Geometry: see drawing. Coordinates: mm, zero at the bounding-box minimum. A direction names the side the tool comes from. Round coordinates to 2 decimals unless told otherwise and drop trailing zeros. Order: outer loops, then holes, each group sorted by start corner. A loop starts at its lowest first (then second) coordinate and runs counter-clockwise, first axis right, second up. Notation, with made-up numbers: (31, -31.75) - (74, -31.75) arc R11 ccw to (74, -16.75) - close; hole circle Ø1 at (56.25, 22.5). An arc over 180 degrees is marked (long way). Put each result on its own line as item: value. Start each with the question number.
1) Section B-B on y = 9.25. Output: boundary loops of the cut face in (x, z) (1 decimal), then the cut area to 3 significant figures.
2) Mould query, pull axis X, two halves, no side actions, for the marked faces 6, 7 and 8. Classes: +X half, -X half, draft (parallel to the pull), parting line (faces both ways), or undercut.
3) Contact query for flat-ended pins moving along their axis: P1, Ø11, axis at x = 5.5, z = 24.5, coming from the +Y side; P2, Ø1, axis at y = 16, z = 28.5, coming from the -X side; P3, Ø7.5, axis at x = 8, y = 6.5, coming from the -Z side. Output: stop coordinate, or through.
4) Line query: probe 1 along X at (y, z) = (4.35, 25.6); probe 2 along X at (y, z) = (14, 48.5); probe 3 along Z at (x, y) = (81, 2.4). Output: solid intervals per line, ascending. Write a range as [from, to].
5) Section A-A on z = 30. Output: boundary loops of the cut face in (x, y).
6) Access query for the marked faces 1, 2, 3, 4 and 5. Directions: +Z, -Z, +X, -X, +Y, -Y. A direction counts if a zero-diameter tool reaches every point of the face in a straight line with its end or side. Return the directions, or none.
7) Section C-C on y = 21.75. Output: boundary loops of the cut face in (x, z).
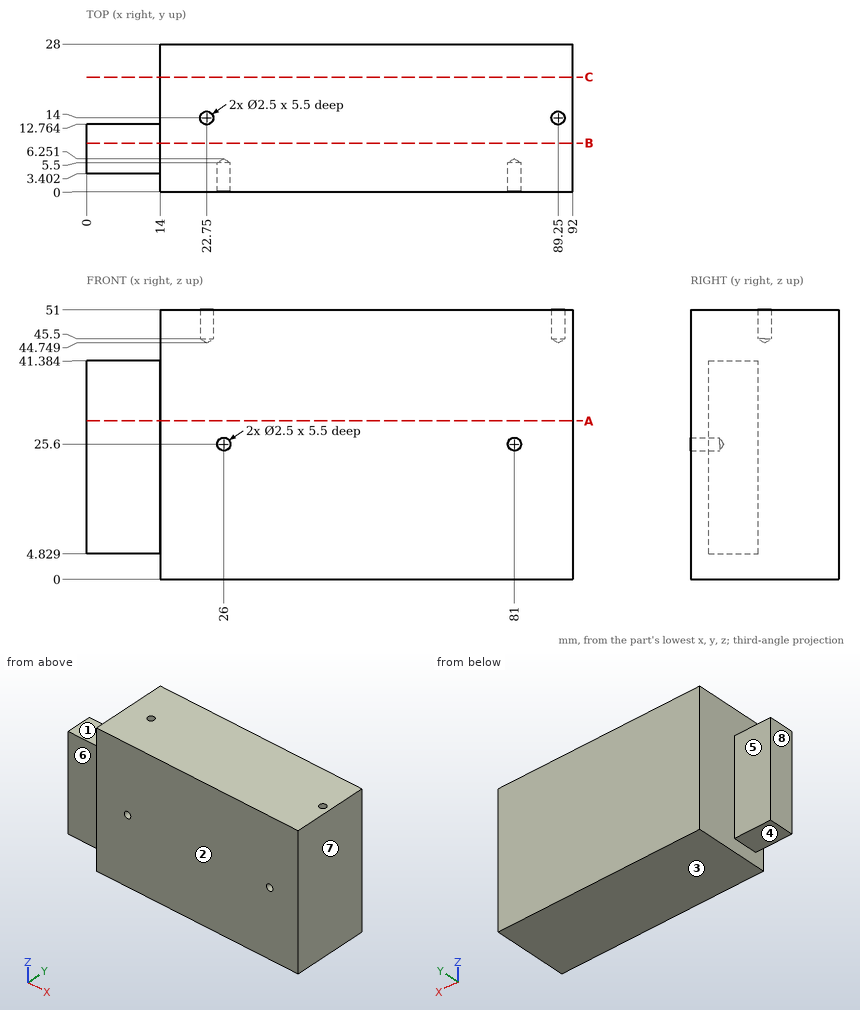
Answer sheet:
1. outline: (0, 4.8) - (14, 4.8) - (14, 0) - (92, 0) - (92, 51) - (14, 51) - (14, 41.4) - (0, 41.4) - close
1. area: 4,490 mm^2
2. face 6: draft
2. face 7: +X half
2. face 8: -X half
3. P1: y = 12.76
3. P2: x = 14
3. P3: z = 4.83
4. probe 1: [0, 24.75], [27.25, 79.75], [82.25, 92]
4. probe 2: [14, 21.5], [24, 88], [90.5, 92]
4. probe 3: [0, 24.35], [26.85, 51]
5. outline: (0, 3.4) - (14, 3.4) - (14, 0) - (92, 0) - (92, 28) - (14, 28) - (14, 12.76) - (0, 12.76) - close
6. face 1: +Z, -X, +Y, -Y
6. face 2: +Z, -Z, +X, -X, -Y
6. face 3: -Z, +X, -X, +Y, -Y
6. face 4: -Z, -X, +Y, -Y
6. face 5: +Z, -Z, -X, +Y
7. outline: (14, 0) - (92, 0) - (92, 51) - (14, 51) - close
